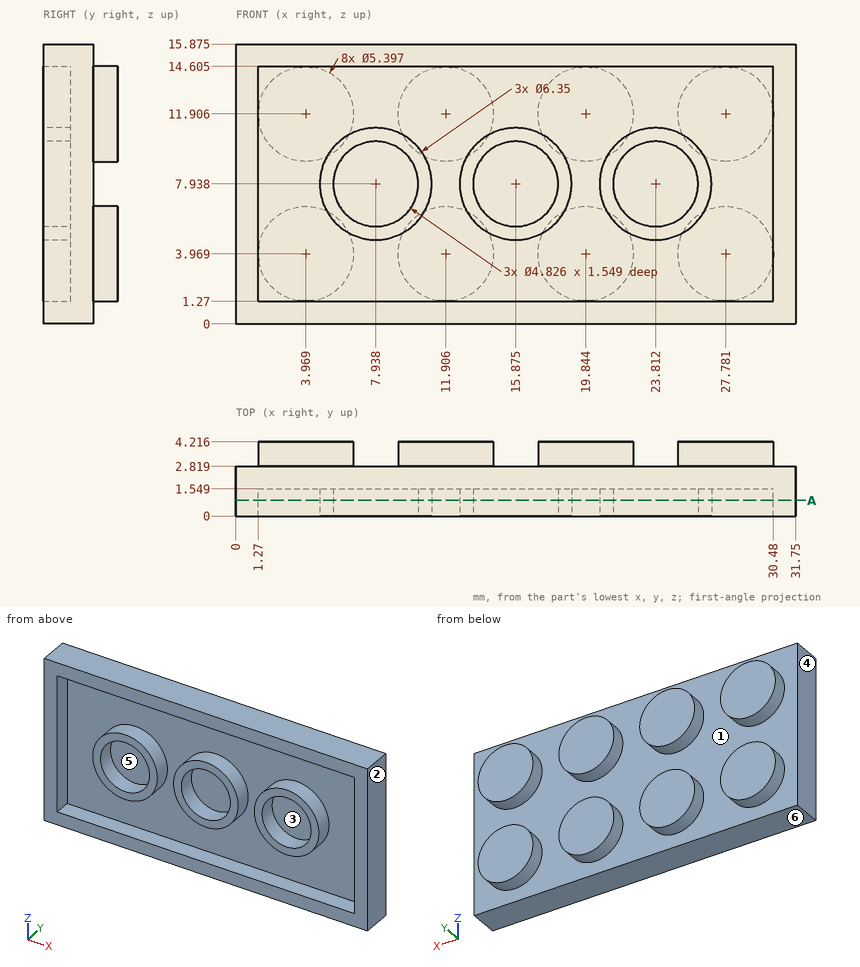
The figure shows three views and two pictorial views of one solid part (mm, origin at its lowest corner). Answer the questions. A direction names the side the tool comes from. Give positions to 0.01 mm unless a question says otherwise; leave off trailing zeros. One line per item, written item: value. Start each with the question number.
(1) Determine the mould class of the marked faces 4, 5 and 6 for opening direction Z: pulls with the +Z half, pulls with the -Z half, needs draft (parallel to the pull), parting line crosses it, or undercut.
(2) A tool of negligible diameter and unlimited length cuts with its end or side. For the marked faces 1, 2 and 3, from which of +Z, -Z, +X, -X, +Y, -Y can it reach the whole face along a straight path? Write none if from no direction.
(3) Find the intervals of material crossed by line 1 (Z direction, x = 9.5, y = 1.5) (1 decimal); line 2 (X direction, y = 0.9, z = 11.75); line 3 (Z direction, x = 29.5, y = 0.45) (1 decimal), in increasing order.
(4) Find section A-A (y = 0.9). Give the number of separate pieces and of enclosed holes in the cut face.
(5) Flat-ended cylindrical pins translate along their axes: pin 1 Ø2.5 at (x, z) = (7, 7.5) entering from -Y; pin 2 Ø5.5 at (x, z) = (7.94, 7.94) entering from +Y. Find the tip coordinate at first contact, or state that the pin passes through.
Results below:
1. face 4: needs draft
1. face 5: undercut
1. face 6: pulls with the -Z half
2. face 1: +Y
2. face 2: +Z, -Z, +X, +Y, -Y
2. face 3: -Y
3. line 1: z = 0 to 1.3, 5.2 to 6.1, 9.8 to 10.7, 14.6 to 15.9
3. line 2: x = 0 to 1.27, 30.48 to 31.75
3. line 3: z = 0 to 1.3, 14.6 to 15.9
4. separate pieces: 4
4. enclosed holes: 4
5. pin 1: stops at y = 1.55
5. pin 2: stops at y = 2.82
